```python
from build123d import *

# Parameters (mm, degrees)
SKETCH1_W           = 50
SKETCH1_H           = 50
BOSS_EXTRUDE1_DEPTH = 25
SKETCH2_R           = 3.15
BOSS_EXTRUDE2_DEPTH = 25
SKETCH3_W           = 5
SKETCH3_H           = 5
CUT_EXTRUDE2_DEPTH  = 6


with BuildPart() as part:
    # Sketch1 → Boss-Extrude1 (new body)
    with BuildSketch(Plane(origin=(0, 0, 0), x_dir=(1, 0, 0), z_dir=(0, 1, 0))):
        Rectangle(SKETCH1_W, SKETCH1_H)
    extrude(amount=BOSS_EXTRUDE1_DEPTH)

    # Sketch2 → Boss-Extrude2 (add)
    with BuildSketch(Plane(origin=(0, 25, 0), x_dir=(1, 0, 0), z_dir=(0, 1, 0))):
        Circle(SKETCH2_R)
    extrude(amount=BOSS_EXTRUDE2_DEPTH)

    # Sketch3 → Cut-Extrude2 (cut)
    with BuildSketch(Plane.ZY.offset(25)):
        with Locations((0, 12.5)):
            Rectangle(SKETCH3_W, SKETCH3_H)
    extrude(amount=-CUT_EXTRUDE2_DEPTH, mode=Mode.SUBTRACT)


solid = part.part
```
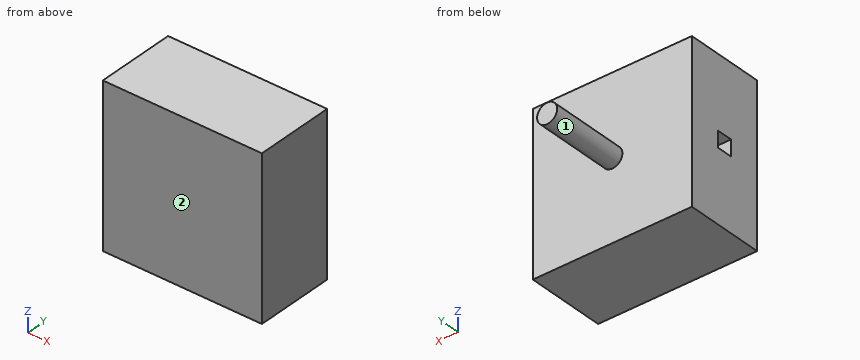
CAD build for the part. Positions are in the model's coordinates, mm. Face numbers are marked on the shaded views. A direction names the side the tool comes from. Coordinates: 2 decimals unless noted, no trailing zeros. Write each loop counter-clockwise with the first axis right and the second up, starting at its lowest first coordinate (ties: lowest second). Pieces come first, ordered by that corner, then holes. Notation, with made-up numbers: (14, -29.5) -> (18, -29.5) arc R24 cw to (18, 3.5) -> close; hole circle Ø2 at (0, -12.75). An arc over 180 degrees is marked (long way). Use CSV: the item, a comma, the result in double quotes. Start each with the question number.
Item 1: Drop flat-ended pins along their axis: P1, Ø2.5, axis at y = 11.5, z = 0.5, coming from the -X side; P2, Ø1.5, axis at x = 3.5, z = 13, coming from the -Y side; P3, Ø2.5, axis at x = -23, z = 0, coming from the +Y side. Give the stop position or say it passes through.
Item 2: Band-saw the part on B-B, the plane z = 0. Write the cut outline in (x, y), plus the area to 3 significant figures.
Item 3: Band-saw the part on A-A, the plane x = 0. Write the cut outline in (y, z), plus the area to 3 significant figures.
Item 4: Wall check: probe 1 along Y at (x, z) = (-0.5, 13); probe 2 along Z at (x, y) = (1, 34.5). Give the ranges that are in metal, low to high.
Item 5: Band-saw the part on D-D, the plane z = 5. Write the cut outline in (x, y).
Item 6: Tool access for the marked faces 1 and 2: list every direction of +Z, -Z, +X, -X, +Y, -Y with a clear straight run to the whole face (end or side of a thin tool).
Item 7: Band-saw the part on C-C, the plane y = 44. Write the cut outline in (x, z), plus the area to 3 significant figures.
Response values:
1,P1,"stops at x = -19"
1,P2,"stops at y = 0"
1,P3,"stops at y = 25"
2,outline,"(-25, 0) -> (25, 0) -> (25, 25) -> (3.15, 25) -> (3.15, 50) -> (-3.15, 50) -> (-3.15, 25) -> (-25, 25) -> (-25, 15) -> (-19, 15) -> (-19, 10) -> (-25, 10) -> close"
2,area,"1,380 mm2"
3,outline,"(0, -25) -> (25, -25) -> (25, -3.15) -> (50, -3.15) -> (50, 3.15) -> (25, 3.15) -> (25, 25) -> (0, 25) -> close"
3,area,"1,410 mm2"
4,probe 1,"y = 0 to 25"
4,probe 2,"z = -2.99 to 2.99"
5,outline,"(-25, 0) -> (25, 0) -> (25, 25) -> (-25, 25) -> close"
6,face 1,"+Y"
6,face 2,"+Z, -Z, +X, -X, -Y"
7,outline,"circle Ø6.3 at (0, 0)"
7,area,"31.2 mm2"
